Autodesk Inventor part; units mm, degrees
ref_plane "YZ Plane" through (0, 0, 0) normal (1, 0, 0) x (0, 1, 0)
ref_plane "XZ Plane" through (0, 0, 0) normal (0, 1, 0) x (-1, 0, 0)
ref_plane "XY Plane" through (0, 0, 0) normal (0, 0, 1) x (1, 0, 0)
sketch "Sketch1" plane through (0, 0, 0) normal (1, 0, 0) x (0, 1, 0)
  line L0 (-1.185, -12.92) -> (1.185, -12.92)
  line L1 (1.185, -12.92) -> (1.185, 12.92)
  line L2 (1.185, 12.92) -> (-1.185, 12.92)
  line L3 (-1.185, 12.92) -> (-1.185, -12.92)
  line L4 (-1.185, -12.92) -> (1.185, 12.92) construction
  line L5 (1.185, -12.92) -> (-1.185, 12.92) construction
  point P0 (0, 0)
  dimension "d0" = 2.37
  dimension "d1" = 25.84
extrude "Extrusion1" add sketch "Sketch1" along normal blind 8.43
sketch "Sketch2" plane through (8.43, 0, 0) normal (1, 0, 0) x (0, 0, -1)
  line L0 (12.92, -1.185) -> (12.92, 1.185)
  line L1 (12.92, 1.185) -> (-12.92, 1.185)
  line L2 (-12.92, 1.185) -> (-12.92, -1.185)
  line L3 (-12.92, -1.185) -> (12.92, -1.185)
  circle A0 centre (-11.47, 0) radius 0.375
  point P0 (0, 0)
  dimension "d4" = 0.75
  dimension "d5" = 1.45
extrude "Extrusion2" add sketch "Sketch2" along normal blind 11.15 contours A0
sketch "Sketch3" plane through (0, 0, 0) normal (-1, 0, 0) x (0, 0, 1)
  circle A0 centre (11.47, 0) radius 0.375
  point P0 (0, 0)
extrude "Extrusion3" cut sketch "Sketch3" against normal blind 7
pattern_linear "Rectangular Pattern1" count 10 spacing 2.54 along (0, 0, -1) of "Extrusion2", "Extrusion3"
ref_plane "Work Plane1" through (0, -1.185, 0) normal (0, 0, 1) x (1, 0, 0)
ref_plane "Work Plane3" through (0, 0, 12.92) normal (0, 1, 0) x (1, 0, 0)
properties part number "00_electricpin_2.54_10x"
For this review, take the finished solid that the model builds, in its own axes (mm). Coordinates: 2 decimals unless noted, no trailing zeros. Loops run counter-clockwise (first coordinate to the right, second up) from the corner with the lowest first, then second, coordinate; pieces in that order, holes last. Notation, with made-up numbers: (6, 53.5) -> (27, 53.5) arc R10 cw to (27, 70.5) -> close; hole circle Ø3 at (-10.5, 75). An arc over 180 degrees is marked (long way). Write each question's results on one line, items separated by ' | '.
Q1. Add section B-B, the plane z = -3.77. State the section outline as (x, y) points (3 decimals).
Taken from the geometry:
outline: (0, -1.185) -> (8.43, -1.185) -> (8.43, -0.375) -> (19.58, -0.375) -> (19.58, 0.375) -> (8.43, 0.375) -> (8.43, 1.185) -> (0, 1.185) -> (0, 0.375) -> (7, 0.375) -> (7, -0.375) -> (0, -0.375) -> close
Q2. Add section A-A, the plane x = 9.5. Count the separate pieces of the cut face and the enclosed holes in it, then the cut area to 3 significant figures.
Taken from the geometry:
separate pieces: 10 | enclosed holes: 0 | area: 4.42 mm²
Q3. Mouldability with a two-part tool opening along Z and no side actions: class faces 1 (the flat face through (4, 0, 12.92)), 2 (the flat face through (0, 0, 0)), 3 (the flat face through (4, 0, -12.92)), 4 (the flat face through (8.43, 0, 0)) as +Z half, -Z half, draft (parallel to the pull), parting line (faces both ways), or undercut.
Taken from the geometry:
face 1: +Z half | face 2: draft | face 3: -Z half | face 4: undercut
Q4. For pin 1 Ø2 at (x, z) = (13.5, 10) entering from +Y, flat-tipped, find the tip position at first contact; note if it passes through.
Taken from the geometry:
pin 1: y = 0.37
Q5. To check wall thickness, follow line 1 along X through (y, z) = (-0.35, -1); line 2 along Y through (x, z) = (4, -6.31) (3 decimals); line 3 along Y through (x, z) = (6.75, -6) (3 decimals). State the ranges of each line that lie inside material, in increasing order. Write a range as [from, to].
Taken from the geometry:
line 1: [0, 8.43] | line 2: [-1.185, -0.375], [0.375, 1.185] | line 3: [-1.185, -0.211], [0.211, 1.185]
Q6. Add section C-C, the plane y = -0.85. State the section outline as (x, z) points.
Taken from the geometry:
outline: (0, -12.92) -> (8.43, -12.92) -> (8.43, 12.92) -> (0, 12.92) -> close
Q7. Add section D-D, the plane z = -10.25. State the section outline as (x, y) points (3 decimals).
Taken from the geometry:
outline: (0, -1.185) -> (8.43, -1.185) -> (8.43, 1.185) -> (0, 1.185) -> close
